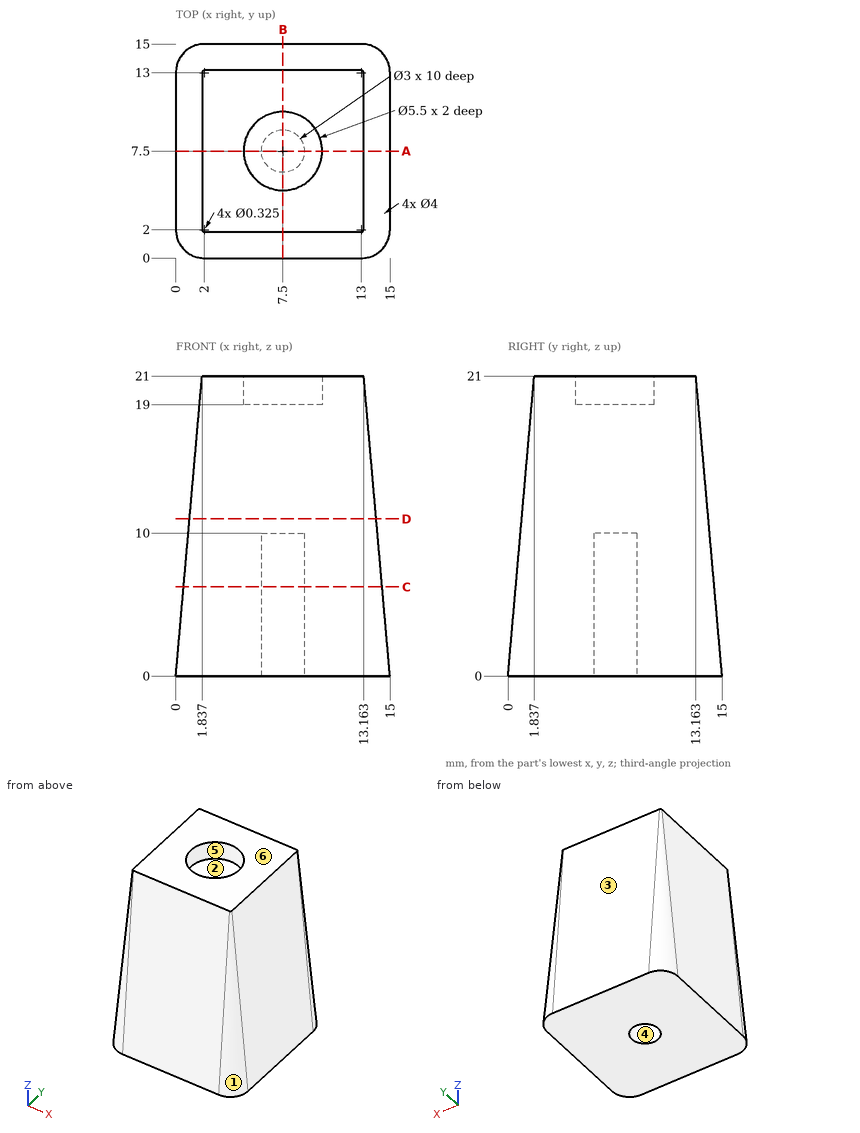
Part print with two shaded views. Sizes in mm from the minimum x, y, z corner. A direction names the side the tool comes from. Round coordinates to 2 decimals unless told otherwise and drop trailing zeros. Write each loop counter-clockwise with the first axis right and the second up, starting at its lowest first coordinate (ties: lowest second). Pieces come first, ordered by that corner, then holes. Notation, with made-up numbers: M -7,-37.75 L 48,-37.75 A19 cw 48,-1.75 Z; hole C -39.75,44 d5. An arc over 180 degrees is marked long. Put each result on its own line as item: value. Start each with the question number.
1) Saw through at D-D, the plane z = 11. Write the cut outline in (x, y) (1 decimal), and give its area (3 significant figures).
2) Pull direction X, two halves, no side cores. Call the marked faces 1, 2 and 3: pulls with the +X half, pulls with the -X half, needs draft (parallel to the pull), parting line crosses it, or undercut.
3) Saw through at C-C, the plane z = 6.25. Write the cut outline in (x, y).
4) Drill centre lines: probe 1 along Y at (x, z) = (9.75, 19.75) (1 decimal); probe 2 along Z at (x, y) = (8.5, 5.5); probe 3 along Y at (x, z) = (7.5, 20.2). Where is each one in solid material? Low to high. Write a range as [from, to].
5) Pin check, flat tips, straight feed: pin 1 Ø4 at (x, z) = (9, 10.5) entering from -Y; pin 2 Ø1.5 at (y, z) = (5.5, 10.5) entering from +X; pin 3 Ø8 at (y, z) = (5.5, 7) entering from -X. Stop position of each tip, or through.
6) 3-axis set-ups, long thin cutter, end or side, ignore diameter. For the marked faces 4, 5 and 6: which of +Z, -Z, +X, -X, +Y, -Y reach the whole face in a straight line?
7) Saw through at A-A, the plane y = 7.5. Write the cut outline in (x, z).
Resolved:
1. outline: M 1,2 A1 ccw 2,1 L 13,1 A1 ccw 14,2 L 14,13 A1 ccw 13,14 L 2,14 A1 ccw 1,13 Z
1. area: 170 mm²
2. face 1: pulls with the +X half
2. face 2: undercut
2. face 3: needs draft
3. outline: M 0.55,2 A1.45 ccw 2,0.55 L 13,0.55 A1.45 ccw 14.45,2 L 14.45,13 A1.45 ccw 13,14.45 L 2,14.45 A1.45 ccw 0.55,13 Z; hole C 7.5,7.5 d3
4. probe 1: [1.7, 5.9], [9.1, 13.3]
4. probe 2: [0, 19]
4. probe 3: [1.77, 4.75], [10.25, 13.23]
5. pin 1: y = 0.74
5. pin 2: x = 14.15
5. pin 3: x = 0.26
6. face 4: -Z
6. face 5: +Z
6. face 6: +Z, +X, -X, +Y, -Y
7. outline: M 0,0 L 6,0 L 6,10 L 9,10 L 9,0 L 15,0 L 13.16,21 L 10.25,21 L 10.25,19 L 4.75,19 L 4.75,21 L 1.84,21 Z
